CAD build for the part. Positions are in the model's coordinates, mm. Coordinates: 2 decimals unless noted, no trailing zeros. Order: outer loops, then holes, each group sorted by start corner. A loop starts at its lowest first (then second) coordinate and runs counter-clockwise, first axis right, second up. Notation, with made-up numbers: M 81.5,-4.75 L 111.5,-4.75 A34 ccw 111.5,28.25 Z; hole C -22,56.5 d2. An arc over 180 degrees is marked long. Write item = value, one per line.
Autodesk Fusion 360 part; units mm, degrees
sketch "Sketch1" plane through (0, 0, 0) normal (0, 1, 0) x (1, 0, 0)
  circle A0 centre (0, 0) radius 5
  circle A1 centre (0, 0) radius 2.5
  dimension "d1" = 10
  dimension "d2" = 5
sketch "Sketch2" plane through (0, 0, 0) normal (0, 1, 0) x (1, 0, 0)
  circle A0 centre (0, 0) radius 5
  circle A1 centre (0, 0) radius 4
  dimension "d5" = 10
  dimension "d6" = 8
sketch "Sketch3" plane through (0, 0, 0) normal (0, 1, 0) x (1, 0, 0)
  circle A0 centre (0, 0) radius 5.15
  circle A1 centre (0, 0) radius 2.85
  dimension "d9" = 10.3
  dimension "d10" = 5.7
extrude "Extrude3" add sketch "Sketch3" along normal blind 1
move_face "OffsetFaces1" offset -0.05 1 faces at (2.8465, 0.6667, 0.1421)
sketch "Sketch4" plane through (0, 1, 0) normal (0, 1, 0) x (-1, 0, 0)
  circle A0 centre (0, 0) radius 2.9
  circle A1 centre (0, 0) radius 5.15
  circle A2 centre (0, 0) radius 3.4
  dimension "d14" = 6.8
extrude "Extrude4" cut sketch "Sketch4" against normal blind 0.15 contours A2
move_face "OffsetFaces2" offset -0.1 1 faces at (2.8964, 0.5667, 0.1446)
move_face "OffsetFaces3" offset 0.05 1 faces at (2.9963, 0.2833, -0.1495)
move_face "OffsetFaces4" offset -0.07 1 faces at (-3.2264, 0.85, -0.3155)
move_face "OffsetFaces5" offset -0.05 1 faces at (-3.3958, 0.8533, -0.1695)
move_face "OffsetFaces6" offset -0.3 1 faces at (-3.4457, 0.8533, -0.172)
equation "d6 = 10 mm - 2 mm"
equation "d10 = 10.3 mm - ( 2.3 * 2 ) * 1 mm"
equation "d14 = 5.800 mm + 1 mm"
(1) Slice it at A-A, the plane x = 0. Write the cut outline in (y, z), then the cut area to 3 significant figures.
Evaluation:
outline = M 0,-5.15 L 1,-5.15 L 1,-3.75 L 0.78,-3.75 L 0.78,-2.95 L 0,-2.95 Z; M 0,2.95 L 0.78,2.95 L 0.78,3.75 L 1,3.75 L 1,5.15 L 0,5.15 Z
area = 4.05 mm²
(2) Pin check, flat tips, straight feed: pin 1 Ø4 at (x, z) = (-1, 1) entering from +Y; pin 2 Ø5 at (x, z) = (1, 0.5) entering from -Y. Stop position of each tip, or through.
Evaluation:
pin_1 = 0.78
pin_2 = 0
(3) Pull direction Z, two halves, no side cores. Call faces 1 (the face through (4.91, 0.49, 1.55)), 2 (the face through (2.2, 0, 2.2)), 3 (the face through (3, 0.78, -1)): +Z half, -Z half, draft (parallel to the pull), parting line (faces both ways), or undercut.
Evaluation:
face_1 = parting line
face_2 = draft
face_3 = undercut
(4) Slice it at C-C, the plane y = 0.6. Write the cut outline in (x, z), then the cut area to 3 significant figures.
Evaluation:
outline = C 0,0 d10.3; hole C 0,0 d5.9
area = 56.0 mm²
(5) Slice it at D-D, the plane x = -3.5. Write the cut outline in (y, z), then the cut area to 3 significant figures.
Evaluation:
outline = M 0,-3.78 L 1,-3.78 L 1,-1.35 L 0.78,-1.35 L 0.78,1.35 L 1,1.35 L 1,3.78 L 0,3.78 Z
area = 6.96 mm²
(6) Slice it at B-B, the plane z = 0. Write the cut outline in (x, y).
Evaluation:
outline = M -5.15,0 L -2.95,0 L -2.95,0.78 L -3.75,0.78 L -3.75,1 L -5.15,1 Z; M 2.95,0 L 5.15,0 L 5.15,1 L 3.75,1 L 3.75,0.78 L 2.95,0.78 Z
(7) Wall check: line 1 (Z direction, x = 0, y = 0.2); line 2 (Z direction, x = 0, y = 0.9); line 3 (X direction, y = 0.9, z = 2.25). Give the ranges that are in metal, low to high. Write a range as from..to.
Evaluation:
line_1 = -5.15..-2.95, 2.95..5.15
line_2 = -5.15..-3.75, 3.75..5.15
line_3 = -4.63..-3, 3..4.63
